Autodesk Inventor part; units mm, degrees
ref_plane "YZ Plane" through (0, 0, 0) normal (1, 0, 0) x (0, 1, 0)
ref_plane "XZ Plane" through (0, 0, 0) normal (0, 1, 0) x (-1, 0, 0)
ref_plane "XY Plane" through (0, 0, 0) normal (0, 0, 1) x (1, 0, 0)
sketch "Sketch1" plane through (0, 0, 0) normal (0, 1, 0) x (-1, 0, 0)
  circle A0 centre (0, 0) radius 2.413
  line L0 (4.7625, -2.7496) -> (0, -5.4993)
  line L1 (0, -5.4993) -> (-4.7625, -2.7496)
  line L2 (-4.7625, -2.7496) -> (-4.7625, 2.7496)
  line L3 (-4.7625, 2.7496) -> (0, 5.4993)
  line L4 (0, 5.4993) -> (4.7625, 2.7496)
  line L5 (4.7625, 2.7496) -> (4.7625, -2.7496)
  dimension "d0" = 4.826
  dimension "d1" = 9.525
extrude "Extrusion1" add sketch "Sketch1" along normal blind 5.1562
properties part number "10-32 nut"
Design review of the part built by this model. Coordinates are the model's own, in mm. Coordinates: 2 decimals unless noted, no trailing zeros. Write each loop counter-clockwise with the first axis right and the second up, starting at its lowest first coordinate (ties: lowest second). Pieces come first, ordered by that corner, then holes. Notation, with made-up numbers: (18, 18) -> (58, 18) arc R9 ccw to (58, 25) -> close; hole circle Ø11 at (21.5, 38.25). An arc over 180 degrees is marked (long way). Write each question's results on one line, items separated by ' | '. Start each with the question number.
(1) Take a section at B-B on y = 2.45. Write out the cut boundary in (x, z), and give its area (3 significant figures).
(2) For line 1 along X through (y, z) = (4.8, 1); line 2 along X through (y, z) = (2.5, 0.25); line 3 along Z through (x, y) = (-3.25, 1.1), list the stretches that pass through material, from the lowest coordinate up. Write a range as from..to.
(3) Take a section at A-A on z = 0. Write out the cut boundary in (x, y), and give its area (3 significant figures).
(4) Take a section at D-D on z = 3. Write out the cut boundary in (x, y), and give its area (3 significant figures).
(5) The part is to be moulded in two halves that separate along Z. For faces 1 (the face through (4.762, 3, 0)), 2 (the face through (2.348, 2.542, -4.144)), 3 (the face through (1.915, 2.542, 1.468)), say which applies: pulls with the +Z half, pulls with the -Z half, needs draft (parallel to the pull), parting line crosses it, or undercut.
(6) Take a section at C-C on x = -0.75. Write out the cut boundary in (y, z), and give its area (3 significant figures).
Results found:
1) outline: (-4.76, -2.75) -> (0, -5.5) -> (4.76, -2.75) -> (4.76, 2.75) -> (0, 5.5) -> (-4.76, 2.75) -> close; hole circle Ø4.83 at (0, 0) | area: 60.3 mm2
2) line 1: x = -4.76..-2.2, 2.2..4.76 | line 2: x = -4.76..-2.4, 2.4..4.76 | line 3: z = -3.62..3.62
3) outline: (-4.76, 0) -> (-2.41, 0) -> (-2.41, 5.16) -> (-4.76, 5.16) -> close; (2.41, 0) -> (4.76, 0) -> (4.76, 5.16) -> (2.41, 5.16) -> close | area: 24.2 mm2
4) outline: (-4.33, 0) -> (4.33, 0) -> (4.33, 5.16) -> (-4.33, 5.16) -> close | area: 44.6 mm2
5) face 1: needs draft | face 2: pulls with the -Z half | face 3: undercut
6) outline: (0, -5.07) -> (5.16, -5.07) -> (5.16, -2.29) -> (0, -2.29) -> close; (0, 2.29) -> (5.16, 2.29) -> (5.16, 5.07) -> (0, 5.07) -> close | area: 28.6 mm2
